```python
from build123d import *

# Parameters (mm, degrees)
SKETCH1_R           = 1.5875
BOSS_EXTRUDE2_DEPTH = 0.79375


with BuildPart() as part:
    # Sketch1 → Boss-Extrude2 (new, symmetric)
    with BuildSketch(Plane(origin=(0, 0, 0), x_dir=(1, 0, 0), z_dir=(0, 1, 0))):
        with BuildLine():
            Line((13.7, 4.133736316), (-13.7, 4.133736316))
            ThreePointArc((-13.7, 4.133736316), (-17.833736316, 0), (-13.7, -4.133736316))
            Line((-13.7, -4.133736316), (13.7, -4.133736316))
            ThreePointArc((13.7, -4.133736316), (17.833736316, 0), (13.7, 4.133736316))
        make_face()
        with Locations(Location((13.7, 0, 0), (0, 0, 270))):
            Circle(SKETCH1_R, mode=Mode.SUBTRACT)
        with Locations(Location((-13.7, 0, 0), (0, 0, 270))):
            Circle(SKETCH1_R, mode=Mode.SUBTRACT)
        with BuildLine():
            Line((9.249344571, -1.633736316), (-9.249344571, -1.633736316))
            ThreePointArc((-9.249344571, -1.633736316), (-9.307422945, 0), (-9.249344571, 1.633736316))
            Line((-9.249344571, 1.633736316), (9.249344571, 1.633736316))
            ThreePointArc((9.249344571, 1.633736316), (9.307422945, 0), (9.249344571, -1.633736316))
        make_face(mode=Mode.SUBTRACT)
    extrude(amount=BOSS_EXTRUDE2_DEPTH, both=True)


solid = part.part
```
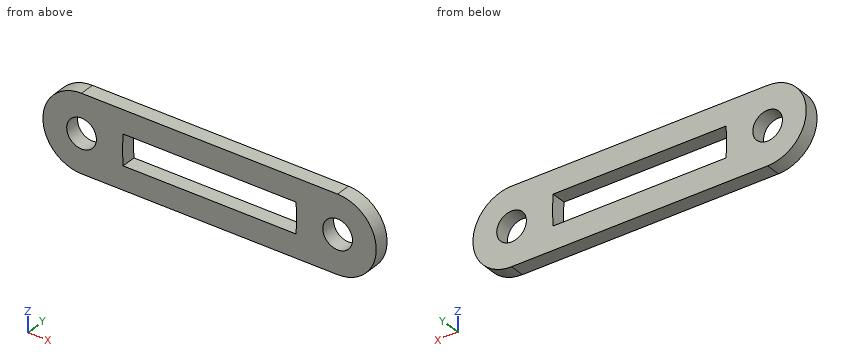
Input: part model. Units: mm. Frame: model coordinates. Coordinates: 2 decimals unless noted, no trailing zeros. Loops run counter-clockwise (first coordinate to the right, second up) from the corner with the lowest first, then second, coordinate; pieces in that order, holes last. Notation, with made-up numbers: M 64.25,-34.75 L 105.25,-34.75 A7 ccw 105.25,-25.75 Z; hole C 16.5,-2.5 d2. An arc over 180 degrees is marked long. Use a Markdown table: item, result. Add a question column.
1) Section C-C, the plane y = -0.15. Return the cut outline in (x, z) (1 decimal).
2) Pin query (flat end, axial travel): P1, Ø1, axis at x = 0.5, z = 1, coming from the +Y side. Return the tip coordinate at first contact, or that it passes through.
3) Section D-D, the plane x = 14. Return the cut outline in (y, z), plus the area to 3 significant figures.
4) Line query: L1, parallel to X at y = -0.25, z = 0; L2, parallel to Z at x = -0.5, y = -0.4; L3, parallel to X at y = 0.4, z = -0.75. Output: solid intervals per line, ascending. Write a range as from..to.
5) Section A-A, the plane z = 0. Return the cut outline in (x, y), plus the area to 3 significant figures.
6) Section B-B, the plane x = -1.5. Return the cut outline in (y, z).
Answer below:
| question | item | result |
|---|---|---|
| 1 | outline | M -13.7,-4.1 L 13.7,-4.1 A4.1 ccw 13.7,4.1 L -13.7,4.1 A4.1 ccw Z; hole C -13.7,0 d3.2; hole M -9.2,-1.6 L 9.2,-1.6 A23 ccw 9.2,1.6 L -9.2,1.6 A23 ccw Z; hole C 13.7,0 d3.2 |
| 2 | P1 | through |
| 3 | outline | M -0.79,-4.12 L 0.79,-4.12 L 0.79,-1.56 L -0.79,-1.56 Z; M -0.79,1.56 L 0.79,1.56 L 0.79,4.12 L -0.79,4.12 Z |
| 3 | area | 8.14 mm2 |
| 4 | L1 | -17.83..-15.29, -12.11..-9.31, 9.31..12.11, 15.29..17.83 |
| 4 | L2 | -4.13..-1.63, 1.63..4.13 |
| 4 | L3 | -17.77..-15.1, -12.3..-9.3, 9.3..12.3, 15.1..17.77 |
| 5 | outline | M -17.83,-0.79 L -15.29,-0.79 L -15.29,0.79 L -17.83,0.79 Z; M -12.11,-0.79 L -9.31,-0.79 L -9.31,0.79 L -12.11,0.79 Z; M 9.31,-0.79 L 12.11,-0.79 L 12.11,0.79 L 9.31,0.79 Z; M 15.29,-0.79 L 17.83,-0.79 L 17.83,0.79 L 15.29,0.79 Z |
| 5 | area | 17.0 mm2 |
| 6 | outline | M -0.79,-4.13 L 0.79,-4.13 L 0.79,-1.63 L -0.79,-1.63 Z; M -0.79,1.63 L 0.79,1.63 L 0.79,4.13 L -0.79,4.13 Z |
